Geometry check sheet. Reference: the model listing, model coordinates, mm. A direction names the side the tool comes from. Give positions to 0.01 mm unless a question says otherwise; leave off trailing zeros. Loops run counter-clockwise (first coordinate to the right, second up) from the corner with the lowest first, then second, coordinate; pieces in that order, holes last. Notation, with made-up numbers: (-35.5, 82) -> (-29.5, 82) arc R11 cw to (-29.5, 90) -> close; hole circle Ø11 at (-39.5, 82.5). An arc over 180 degrees is marked (long way). Write item = value, one per line.
Autodesk Inventor part; units mm, degrees
ref_plane "Work Plane1" through (0, 11.25, 0) normal (0, 1, 0) x (1, 0, 0)
ref_plane "YZ Plane" through (0, 0, 0) normal (1, 0, 0) x (0, 1, 0)
ref_plane "XZ Plane" through (0, 0, 0) normal (0, 1, 0) x (-1, 0, 0)
sketch "Sketch1" plane through (0, 0, 0) normal (0, 1, 0) x (-1, 0, 0)
  line L0 (-55.26, 33.75) -> (55.26, 33.75)
  line L1 (55.26, 33.75) -> (55.26, -33.75)
  line L2 (55.26, -33.75) -> (-55.26, -33.75)
  line L3 (-55.26, -33.75) -> (-55.26, 33.75)
  line L4 (-55.26, 33.75) -> (55.26, -33.75) construction
  line L5 (55.26, 33.75) -> (-55.26, -33.75) construction
  point P0 (0, 0)
  dimension "d0" = 110.52
  dimension "d1" = 67.5
extrude "Extrusion1" add sketch "Sketch1" along normal blind 3
fillet "Fillet1" radius 5.25 4 edges at (-55.26, 1.5, 33.75) (55.26, 1.5, 33.75) (55.26, 1.5, -33.75) (-55.26, 1.5, -33.75)
sketch "Sketch2" plane through (0, 0, 0) normal (0, -1, 0) x (1, 0, 0)
  arc A0 (-55.26, -28.5) -> (-50.01, -33.75) centre (-50.01, -28.5) ccw construction
  line L0 (50.01, -33.75) -> (-50.01, -33.75) construction
  arc A1 (50.01, -33.75) -> (55.26, -28.5) centre (50.01, -28.5) ccw construction
  line L1 (55.26, 28.5) -> (55.26, -28.5) construction
  arc A2 (55.26, 28.5) -> (50.01, 33.75) centre (50.01, 28.5) ccw construction
  line L2 (-50.01, 33.75) -> (50.01, 33.75) construction
  arc A3 (-50.01, 33.75) -> (-55.26, 28.5) centre (-50.01, 28.5) ccw construction
  line L3 (-55.26, -28.5) -> (-55.26, 28.5) construction
  circle A4 centre (-50.01, 28.5) radius 5.25
  line L4 (-50.01, 33.75) -> (50.01, 33.75) construction
  line L5 (-50.01, 33.75) -> (50.01, 33.75)
  line L6 (-55.26, 28.5) -> (-55.26, -28.5)
  circle A5 centre (-50.01, -28.5) radius 5.25
  line L7 (-50.01, -33.75) -> (50.01, -33.75)
  circle A6 centre (50.01, -28.5) radius 5.25
  line L8 (55.26, 28.5) -> (55.26, -28.5)
  circle A7 centre (50.01, 28.5) radius 5.25
  line L9 (51.01, 35.75) -> (-51.01, 35.75)
  line L10 (-57.26, 29.5) -> (-57.26, -29.5)
  line L11 (-51.01, -35.75) -> (51.01, -35.75)
  line L12 (57.26, -29.5) -> (57.26, 29.5)
  line L13 (57.26, 35.75) -> (-57.26, -35.75) construction
  line L14 (-57.26, 35.75) -> (57.26, -35.75) construction
  arc A8 (-51.01, 35.75) -> (-57.26, 29.5) centre (-51.01, 29.5) ccw
  arc A9 (-57.26, -29.5) -> (-51.01, -35.75) centre (-51.01, -29.5) ccw
  arc A10 (51.01, -35.75) -> (57.26, -29.5) centre (51.01, -29.5) ccw
  arc A11 (57.26, 29.5) -> (51.01, 35.75) centre (51.01, 29.5) ccw
  point P0 (0, 0)
  point P1 (55.26, -28.5)
  point P2 (50.01, 33.75)
  dimension "d5" = 2
  dimension "d6" = 2
  dimension "d7" = 6.25
  dimension "d8" = 6.25
extrude "Extrusion2" add sketch "Sketch2" against normal blind 26
sketch "Sketch3" plane through (55.26, 3, 28.5) normal (-1, 0, 0) x (0, 0, 1)
  line L0 (0, 0) -> (-57, 0) construction
  line L1 (-57, 23) -> (0, 23) construction
  line L2 (-54.5, 0) -> (-27, 0)
  line L3 (-27, 0) -> (-27, 47.408)
  line L4 (-27, 47.408) -> (-54.5, 47.408)
  line L5 (-54.5, 47.408) -> (-54.5, 0)
  line L6 (-62.25, 0) -> (-62.25, 23) construction
  point P0 (-28.5, -3)
  point P1 (-54.5, 23.704)
  point P2 (-40.75, 47.408)
  dimension "d11" = 7.75
  dimension "d12" = 27.5
  dimension "d13" = 24.408
extrude "Extrusion3" add sketch "Sketch3" along normal blind 3
sketch "Sketch4" plane through (0, 3, 0) normal (0, 1, 0) x (1, 0, 0)
  arc A0 (55.26, 28.5) -> (50.01, 33.75) centre (50.01, 28.5) ccw construction
  line L0 (50.01, 33.75) -> (-50.01, 33.75) construction
  line L1 (-50.01, -33.75) -> (50.01, -33.75) construction
  arc A1 (50.01, -33.75) -> (55.26, -28.5) centre (50.01, -28.5) ccw construction
  line L2 (55.26, -28.5) -> (55.26, -1.5) construction
  circle A2 centre (50.01, 28.5) radius 2.5
  circle A3 centre (50.01, -28.5) radius 2.5
  line L3 (47.51, -28.5) -> (47.51, -33.75)
  line L4 (55.26, -26) -> (50.01, -26)
  line L5 (0, 0) -> (0, -21.4582)
  line L6 (0, 0) -> (16.5599, 0)
  line L7 (47.51, 28.5) -> (47.51, 33.75)
  line L8 (55.26, 26) -> (50.01, 26)
  circle A4 centre (-50.01, 28.5) radius 2.5
  circle A5 centre (-50.01, -28.5) radius 2.5
  line L9 (-47.51, -28.5) -> (-47.51, -33.75)
  line L10 (-55.26, -26) -> (-50.01, -26)
  line L11 (-47.51, 28.5) -> (-47.51, 33.75)
  line L12 (-55.26, 26) -> (-50.01, 26)
  line L13 (55.26, 28.5) -> (55.26, -28.5)
  line L14 (50.01, 33.75) -> (5.9104, 33.75)
  arc A6 (55.26, 28.5) -> (50.01, 33.75) centre (50.01, 28.5) ccw
  arc A7 (50.01, -33.75) -> (55.26, -28.5) centre (50.01, -28.5) ccw
  line L15 (50.01, -33.75) -> (5.9104, -33.75)
  line L16 (-55.26, 26) -> (-55.26, 28.5) construction
  arc A8 (-50.01, 33.75) -> (-55.26, 28.5) centre (-50.01, 28.5) ccw construction
  line L17 (-50.01, 33.75) -> (50.01, 33.75) construction
  arc A9 (-55.26, -28.5) -> (-50.01, -33.75) centre (-50.01, -28.5) ccw construction
  line L18 (-55.26, -28.5) -> (-55.26, -1.5) construction
  line L19 (-55.26, 28.5) -> (-55.26, -28.5)
  line L20 (-50.01, 33.75) -> (-5.9104, 33.75)
  arc A10 (-50.01, 33.75) -> (-55.26, 28.5) centre (-50.01, 28.5) ccw
  arc A11 (-55.26, -28.5) -> (-50.01, -33.75) centre (-50.01, -28.5) ccw
  line L21 (-50.01, -33.75) -> (-5.9104, -33.75)
  point P0 (-47.51, 28.5)
  dimension "d16" = 5
  dimension "d17" = 5
extrude "Extrusion4" add sketch "Sketch4" along normal blind 15.25
ref_plane "Work Plane1" through (0, 11.25, 0) normal (0, 1, 0) x (1, 0, 0)
sketch "Sketch5" plane through (0, 3, 0) normal (0, 1, 0) x (1, 0, 0)
  line L0 (-47.51, -33.75) -> (47.51, -33.75) construction
  arc A0 (-55.26, -28.5) -> (-50.01, -33.75) centre (-50.01, -28.5) ccw construction
  line L1 (-47.51, 28.5) -> (-55.26, 28.5)
  line L2 (-55.26, 28.5) -> (-55.26, -28.5)
  line L3 (-55.26, -28.5) -> (-47.51, -28.5)
  line L4 (-47.51, -28.5) -> (-47.51, 28.5)
  line L5 (-7.51, -33.75) -> (-5.51, -33.75)
  line L6 (-5.51, -33.75) -> (-5.51, 28.75)
  line L7 (-5.51, 28.75) -> (-7.51, 28.75)
  line L8 (-7.51, 28.75) -> (-7.51, -33.75)
  line L9 (-1.51, -33.75) -> (0.49, -33.75)
  dimension "d21" = 2
  dimension "d22" = 40
extrude "Extrusion5" add sketch "Sketch5" along normal blind 6
sketch "Sketch6" plane through (0, 3, 0) normal (0, 1, 0) x (1, 0, 0)
  line L0 (55.26, -1.5) -> (52.26, -1.5) construction
  line L1 (52.26, 26) -> (27.26, 26)
  line L2 (27.26, 26) -> (27.26, -1.5)
  line L3 (27.26, -1.5) -> (52.26, -1.5)
  line L4 (52.26, -1.5) -> (52.26, 26)
  line L5 (57.26, -29.5) -> (57.26, 29.5) construction
  point P0 (0, 0)
  point P1 (27.26, 12.25)
  dimension "d29" = 30
extrude "Extrusion6" add sketch "Sketch6" along normal up to surface (15.25 mm away)
sketch "Sketch7" plane through (57.26, 0, 29.5) normal (1, 0, 0) x (0, 0, -1)
  line L0 (59, 0) -> (0, 0) construction
  line L1 (0, 26) -> (59, 26) construction
  line L2 (48.75, 5.5) -> (34.75, 5.5)
  line L3 (34.75, 5.5) -> (34.75, 14.5)
  line L4 (34.75, 14.5) -> (48.75, 14.5)
  line L5 (48.75, 14.5) -> (48.75, 5.5)
  line L6 (48.75, 5.5) -> (34.75, 14.5) construction
  line L7 (34.75, 5.5) -> (48.75, 14.5) construction
  circle A0 centre (41.75, 10) radius 3.5
  line L8 (30.75, 16) -> (52.75, 16)
  line L9 (52.75, 16) -> (52.75, 4)
  line L10 (52.75, 4) -> (30.75, 4)
  line L11 (30.75, 4) -> (30.75, 16)
  line L12 (30.75, 16) -> (52.75, 4) construction
  line L13 (52.75, 16) -> (30.75, 4) construction
  line L14 (52.75, 16) -> (52.75, 26)
  line L15 (55.5, 50.408) -> (55.5, 18.25) construction
  line L16 (55.5, 26) -> (52.75, 26)
  line L17 (28, 26) -> (28, 50.408) construction
  line L18 (28, 26) -> (30.75, 26)
  line L19 (30.75, 16) -> (30.75, 26)
  point P0 (29.5, 0)
  dimension "d32" = 14
  dimension "d33" = 9
  dimension "d34" = 7
  dimension "d35" = 22
  dimension "d36" = 12
  dimension "d37" = 4
extrude "Extrusion7" cut sketch "Sketch7" against normal blind 13 contours L2 L3 L4 L5 | A0 | L8 L9 L10 L11
extrude "Extrusion8" cut sketch "Sketch7" against normal blind 20 contours A0
extrude "Extrusion9" cut sketch "Sketch7" against normal up to surface (10 mm away) from surface at -20 contours L2 L3 L4 L5 | A0
sketch "Sketch8" plane through (0, 3, 0) normal (0, 1, 0) x (1, 0, 0)
  line L0 (55.26, -1.5) -> (27.26, -1.5) construction
  line L1 (47.51, 33.75) -> (-47.51, 33.75) construction
  line L2 (-5.51, 28.75) -> (-5.51, -33.75) construction
  line L3 (-1.51, 25.75) -> (16.49, 25.75)
  line L4 (16.49, 25.75) -> (16.49, -1.75)
  line L5 (16.49, -1.75) -> (-1.51, -1.75)
  line L6 (-1.51, -1.75) -> (-1.51, 25.75)
  line L7 (-3.51, -8.5) -> (31.49, -8.5)
  line L8 (31.49, -8.5) -> (31.49, -27)
  line L9 (31.49, -27) -> (-3.51, -27)
  line L10 (-3.51, -27) -> (-3.51, -8.5)
  line L11 (57.26, -29.5) -> (57.26, 29.5) construction
  line L12 (-4.51, -22.25) -> (3.49, -22.25)
  line L13 (3.49, -22.25) -> (3.49, -13.25)
  line L14 (3.49, -13.25) -> (-4.51, -13.25)
  line L15 (-4.51, -13.25) -> (-4.51, -22.25)
  line L16 (-4.51, -22.25) -> (3.49, -13.25) construction
  line L17 (3.49, -22.25) -> (-4.51, -13.25) construction
  line L18 (25.49, -23.25) -> (31.49, -23.25)
  line L19 (31.49, -23.25) -> (31.49, -12.25)
  line L20 (31.49, -12.25) -> (25.49, -12.25)
  line L21 (25.49, -12.25) -> (25.49, -23.25)
  line L22 (25.49, -23.25) -> (31.49, -12.25) construction
  line L23 (31.49, -23.25) -> (25.49, -12.25) construction
  circle A0 centre (27.49, -22.25) radius 0.75
  point P0 (0, 0)
  point P1 (-0.51, -17.75)
  point P2 (-4.51, -17.75)
  point P3 (-3.51, -17.75)
  point P4 (28.49, -17.75)
  point P5 (31.49, -17.75)
  dimension "d44" = 18
  dimension "d45" = 27.5
  dimension "d46" = 8
  dimension "d48" = 35
  dimension "d49" = 18.5
  dimension "d52" = 7
  dimension "d59" = 2
  dimension "d60" = 4
  dimension "d75" = 1
  dimension "d76" = 9
  dimension "d77" = 8
  dimension "d78" = 11
  dimension "d79" = 6
  dimension "d80" = 1.5
  dimension "d81" = 1
  dimension "d82" = 2
sketch "Sketch9" plane through (55.26, 26, 1.5) normal (0, 0, 1) x (1, 0, 0)
  line L0 (-3, -7.75) -> (-28, -7.75) construction
  line L1 (0, -23) -> (-28, -23) construction
  line L2 (-20, -14.75) -> (-10, -14.75)
  line L3 (-10, -14.75) -> (-10, -17.5)
  line L4 (-10, -17.5) -> (-20, -17.5)
  line L5 (-20, -17.5) -> (-20, -14.75)
  line L6 (2, -22) -> (2, -10) construction
  point P0 (-55.26, -26)
  point P1 (-20, -16.125)
  point P2 (-10, -16.125)
  point P3 (2, -16)
  point P4 (-15, -14.75)
  dimension "d53" = 7
  dimension "d54" = 5.5
  dimension "d55" = 10
  dimension "d56" = 17
extrude "Extrusion10" add sketch "Sketch9" along normal up to surface (32.25 mm away)
sketch "Sketch10" plane through (57.26, 0, 29.5) normal (1, 0, 0) x (0, 0, -1)
  line L0 (12.25, 5.5) -> (18.25, 5.5) construction
  line L1 (12.25, 3.75) -> (18.25, 3.75)
  line L2 (18.25, 7.25) -> (12.25, 7.25)
  arc A0 (12.25, 7.25) -> (12.25, 3.75) centre (12.25, 5.5) ccw
  arc A1 (18.25, 3.75) -> (18.25, 7.25) centre (18.25, 5.5) ccw
  line L3 (3.5, 3) -> (3.5, 18.25) construction
  line L4 (3.5, 3) -> (28, 3) construction
  point P0 (29.5, 0)
  point P1 (15.25, 5.5)
  point P2 (20, 5.5)
  point P3 (10.5, 5.5)
  dimension "d61" = 3.5
  dimension "d62" = 9.5
  dimension "d63" = 7
  dimension "d64" = 0.75
extrude "Extrusion11" cut sketch "Sketch10" against normal blind 10
sketch "Sketch11" plane through (0, 3, 0) normal (0, 1, 0) x (1, 0, 0)
  line L0 (55.26, -26) -> (55.26, -1.5) construction
  line L1 (48.76, -8) -> (55.26, -8)
  line L2 (55.26, -8) -> (55.26, -20.5)
  line L3 (55.26, -20.5) -> (48.76, -20.5)
  line L4 (48.76, -20.5) -> (48.76, -8)
  line L5 (48.76, -8) -> (55.26, -20.5) construction
  line L6 (55.26, -8) -> (48.76, -20.5) construction
  line L7 (45.26, -1.5) -> (45.26, -33.75) construction
  line L8 (48.76, -8) -> (45.26, -8)
  line L9 (45.26, -8) -> (45.26, -6)
  line L10 (45.26, -6) -> (48.76, -6)
  line L11 (48.76, -6) -> (48.76, -8)
  line L12 (48.76, -20.5) -> (45.26, -20.5)
  line L13 (45.26, -20.5) -> (45.26, -22.5)
  line L14 (45.26, -22.5) -> (48.76, -22.5)
  line L15 (48.76, -22.5) -> (48.76, -20.5)
  line L16 (50.01, -26) -> (55.26, -26)
  point P0 (0, 0)
  point P1 (52.01, -14.25)
  point P2 (55.26, -13.75)
  point P3 (55.26, -14.25)
  dimension "d67" = 12.5
  dimension "d68" = 6.5
  dimension "d69" = 2
  dimension "d70" = 2
  dimension "d102" = 11.75
extrude "Extrusion12" cut sketch "Sketch11" against normal blind 2 contours L15 L14 L13 L12 | L8 L9 L10 L11
sketch "Sketch12" plane through (0, 3, 0) normal (0, 1, 0) x (1, 0, 0)
  line L0 (35.26, -1.5) -> (35.26, -33.75) construction
  line L1 (35.26, -1.5) -> (45.26, -1.5)
  line L2 (45.26, -1.5) -> (45.26, -8)
  line L3 (45.26, -8) -> (35.26, -8)
  line L4 (35.26, -8) -> (35.26, -1.5)
  line L5 (35.26, -33.75) -> (45.26, -33.75)
  line L6 (45.26, -33.75) -> (45.26, -20.5)
  line L7 (45.26, -20.5) -> (35.26, -20.5)
  line L8 (35.26, -20.5) -> (35.26, -33.75)
  point P0 (0, 0)
extrude "Extrusion13" add sketch "Sketch12" along normal up to surface (8.25 mm away)
extrude "Extrusion14" cut sketch "Sketch8" against normal blind 1.5 contours L14 L13 L12 L10 | L10 L12 L15 L14 | L8 L18 L21 L20 | A0
extrude "Extrusion15" cut sketch "Sketch8" against normal through all contours A0
sketch "Sketch14" plane through (0, 0, 0) normal (0, -1, 0) x (1, 0, 0)
  arc A0 (51.01, -35.75) -> (57.26, -29.5) centre (51.01, -29.5) ccw
  arc A1 (55.26, 28.5) -> (50.01, 33.75) centre (50.01, 28.5) ccw
  arc A2 (57.26, 29.5) -> (51.01, 35.75) centre (51.01, 29.5) ccw
  arc A3 (-51.01, 35.75) -> (-57.26, 29.5) centre (-51.01, 29.5) ccw
  arc A4 (-50.01, 33.75) -> (-55.26, 28.5) centre (-50.01, 28.5) ccw
  arc A5 (-57.26, -29.5) -> (-51.01, -35.75) centre (-51.01, -29.5) ccw
  arc A6 (-55.26, -28.5) -> (-50.01, -33.75) centre (-50.01, -28.5) ccw
  arc A7 (50.01, -33.75) -> (55.26, -28.5) centre (50.01, -28.5) ccw
  point P0 (0, 0)
hole "Hole2" at (51.01, 0, -29.5) at (-51.01, 0, -29.5) at (-51.01, 0, 29.5) at (51.01, 0, 29.5) direction (0, 1, 0) diameter 3.4 end through all counterbore diameter 7 counterbore depth 4
properties part number "bottom"
Item 1: Gauge pin test, flat ends, axial feed: pin 1 (11 mm diameter, centred on x = 51.01, z = 29.5, fed in from +Y); pin 2 (1.6 mm diameter, centred on y = 10, z = 31.5, fed in from -X); pin 3 (0.9 mm diameter, centred on x = 54, y = 38, fed in from -Z). Record the tip position at first contact, or that the pin passes through.
Answer:
pin_1 = 26
pin_2 = -57.14
pin_3 = -26
Item 2: Section check A-A, the plane y = 22. Record the cut outline in (x, z), plus the area to 3 significant figures.
Answer:
outline = (-57.26, -29.5) arc R6.25 ccw to (-51.01, -35.75) -> (51.01, -35.75) arc R6.25 ccw to (57.26, -29.5) -> (57.26, 29.5) arc R6.25 ccw to (51.01, 35.75) -> (-51.01, 35.75) arc R6.25 ccw to (-57.26, 29.5) -> close; hole (-55.26, -28.5) arc R5.25 ccw to (-50.01, -33.75) -> (50.01, -33.75) arc R5.25 ccw to (55.26, -28.5) -> (55.26, -26) -> (52.26, -26) -> (52.26, 1.5) -> (55.26, 1.5) -> (55.26, 28.5) arc R5.25 ccw to (50.01, 33.75) -> (-50.01, 33.75) arc R5.25 ccw to (-55.26, 28.5) -> close
area = 801 mm^2
Item 3: Draft check along Z on faces 1 (the cylindrical face through (-55.48, 12.82, -33.87)), 2 (the flat face through (-17, 26, -34)), 3 (the flat face through (55.26, 22, -27)). Enter one of: +Z half, -Z half, draft (parallel to the pull), parting line (faces both ways), or undercut.
Answer:
face_1 = -Z half
face_2 = draft
face_3 = undercut
Item 4: Section check D-D, the plane y = 38.5. Record the cut outline in (x, z).
Answer:
outline = (52.26, -26) -> (55.26, -26) -> (55.26, 1.5) -> (52.26, 1.5) -> close
Item 5: Thickness scan on L1, parallel to Z at x = -51.01, y = 10; L2, parallel to X at y = 0.9, z = 29.5; L3, parallel to Z at x = 51.01, y = 15. Record the ranges inside material, lowest first. Write a range as [from, to].
Answer:
L1 = [-35.75, -31.2], [-27.8, -26], [26, 27.8], [31.2, 35.75]
L2 = [-57.26, -54.51], [-47.51, 47.51], [54.51, 57.26]
L3 = [-35.75, -31.2], [-27.8, -23.25], [-1.25, 1.5], [26, 27.8], [31.2, 35.75]
Item 6: Tool access check on faces 4 (the flat face through (51, 10, -1.25)), 5 (the cylindrical face through (-47.905, 2.028, -31.115)), 6 (the flat face through (28, 1.5, 18)). Record the directions out of +Z, -Z, +X, -X, +Y, -Y that give a thin tool (end or side, any length) a straight path to the whole face; none if there is none.
Answer:
face_4 = +X
face_5 = -Y
face_6 = +Y
Item 7: Section check C-C, the plane x = -36. Record the cut outline in (y, z), plus the area to 4 significant figures.
Answer:
outline = (0, -35.75) -> (26, -35.75) -> (26, -33.75) -> (3, -33.75) -> (3, 33.75) -> (26, 33.75) -> (26, 35.75) -> (0, 35.75) -> close
area = 306.5 mm^2
